Here's how the part is built. I have some questions about the finished solid (model axes, mm). A direction names the side the tool comes from. Coordinates: 2 decimals unless noted, no trailing zeros. Loops run counter-clockwise (first coordinate to the right, second up) from the corner with the lowest first, then second, coordinate; pieces in that order, holes last.
from build123d import *

# Parameters (mm, degrees)
SKETCH1_R           = 2.55
BOSS_EXTRUDE1_DEPTH = 8
SKETCH2_R           = 3.175
CUT_EXTRUDE1_DEPTH  = 1
CUT_EXTRUDE2_START  = -1
SKETCH3_R           = 3.175
CUT_EXTRUDE2_DEPTH  = 1
BOSS_EXTRUDE2_DEPTH = 8
SKETCH5_W           = 8
SKETCH5_H           = 56
BOSS_EXTRUDE3_DEPTH = 8
SKETCH6_W           = 4
SKETCH6_H           = 24
CUT_EXTRUDE3_DEPTH  = 8
FILLET2_R           = 4
SKETCH7_R           = 2.55
CUT_EXTRUDE4_DEPTH  = 8
SKETCH8_R           = 3.175
CUT_EXTRUDE5_DEPTH  = 1
CUT_EXTRUDE6_START  = -1
SKETCH9_R           = 3.175
CUT_EXTRUDE6_DEPTH  = 1
FILLET3_R           = 4
FILLET5_R           = 4


# Some blends are built 0.0001 mm under size
with BuildPart() as part:
    # Sketch1 → Boss-Extrude1 (new body)
    with BuildSketch(Plane.YZ):
        Polygon((0, 0), (72, 0), (72, 24), (88, 24), (88, 32), (64, 32), (64, 8), (0, 8), align=None)
        with Locations(Location((12, 4, 0), (0, 0, 270))):
            Circle(SKETCH1_R, mode=Mode.SUBTRACT)
        with Locations(Location((44, 4, 0), (0, 0, 270))):
            Circle(SKETCH1_R, mode=Mode.SUBTRACT)
        with Locations(Location((60, 4, 0), (0, 0, 270))):
            Circle(SKETCH1_R, mode=Mode.SUBTRACT)
        with Locations(Location((68, 28, 0), (0, 0, 270))):
            Circle(SKETCH1_R, mode=Mode.SUBTRACT)
        with Locations(Location((84, 28, 0), (0, 0, 270))):
            Circle(SKETCH1_R, mode=Mode.SUBTRACT)
    extrude(amount=BOSS_EXTRUDE1_DEPTH)

    # Sketch2 → Cut-Extrude1 (cut)
    with BuildSketch(Plane.YZ.offset(8)):
        with Locations(Location((68, 28, 0), (0, 0, 270))):
            Circle(SKETCH2_R)
        with Locations(Location((84, 28, 0), (0, 0, 270))):
            Circle(SKETCH2_R)
        with Locations(Location((12, 4, 0), (0, 0, 270))):
            Circle(SKETCH2_R)
        with Locations(Location((44, 4, 0), (0, 0, 270))):
            Circle(SKETCH2_R)
        with Locations(Location((60, 4, 0), (0, 0, 270))):
            Circle(SKETCH2_R)
    extrude(amount=-CUT_EXTRUDE1_DEPTH, mode=Mode.SUBTRACT)

    # Sketch3 → Cut-Extrude2 (cut)
    with BuildSketch(Plane(origin=(0, 0, 0), x_dir=(0, -1, 0), z_dir=(-1, 0, 0)).offset(CUT_EXTRUDE2_START)):
        with Locations(Location((-12, 4, 0), (0, 0, 270))):
            Circle(SKETCH3_R)
        with Locations(Location((-84, 28, 0), (0, 0, 270))):
            Circle(SKETCH3_R)
        with Locations(Location((-68, 28, 0), (0, 0, 270))):
            Circle(SKETCH3_R)
        with Locations(Location((-60, 4, 0), (0, 0, 270))):
            Circle(SKETCH3_R)
        with Locations(Location((-44, 4, 0), (0, 0, 270))):
            Circle(SKETCH3_R)
    extrude(amount=CUT_EXTRUDE2_DEPTH, mode=Mode.SUBTRACT)

    # Sketch4 → Boss-Extrude2 (add)
    with BuildSketch(Plane.XY.offset(8)):
        with BuildLine():
            Line((0, 0), (0, -4))
            ThreePointArc((0, -4), (0.723391823, -6.294305745), (2.631919427, -7.758770483))
            Line((2.631919427, -7.758770483), (15.787616118, -12.54705249))
            Line((15.787616118, -12.54705249), (18.523777264, -5.029511523))
            Line((18.523777264, -5.029511523), (8, -1.199169847))
            Line((8, -1.199169847), (8, 0))
            Line((8, 0), (0, 0))
        make_face()
    extrude(amount=-BOSS_EXTRUDE2_DEPTH)

    # Sketch5 → Boss-Extrude3 (add)
    with BuildSketch(Plane(origin=(0.550416468, 1.512256816, 0), x_dir=(-0.9396926207859096, 0.34202014332566544, 0), z_dir=(0.3420201433256654, 0.9396926207859095, 0))):
        with Locations((-15.126851056, -4)):
            Rectangle(SKETCH5_W, SKETCH5_H)
    extrude(amount=-BOSS_EXTRUDE3_DEPTH)

    # Sketch6 → Cut-Extrude3 (cut)
    with BuildSketch(Plane(origin=(0.550416468, 1.512256816, 0), x_dir=(-0.9396926207859096, 0.34202014332566544, 0), z_dir=(0.3420201433256654, 0.9396926207859095, 0))):
        with Locations((-17.126851056, -4)):
            Rectangle(SKETCH6_W, SKETCH6_H)
    extrude(amount=-CUT_EXTRUDE3_DEPTH, mode=Mode.SUBTRACT)

    # Fillet2
    # the kernel refuses this fillet: 4 mm, written as the material it adds along each edge
    with BuildSketch(Plane(origin=(8.270075151, -9.810891343, 0), x_dir=(-0.9396926207859096, 0.34202014332566544, 0), z_dir=(0.34202014332566544, 0.9396926207859096, 0))) as fillet2_piece_1_section:
        with BuildLine():
            CenterArc((FILLET2_R, -FILLET2_R), FILLET2_R, 90, 90)
            Line((0, -FILLET2_R), (0, 0))
            Line((0, 0), (FILLET2_R, 0))
        make_face()
    fillet2_piece_1 = extrude(amount=8, mode=Mode.PRIVATE)
    fillet2_piece_1 = split(fillet2_piece_1, bisect_by=Plane(origin=(8, -7.10901072, -0.334730566), z_dir=(-1, 0, 0)), keep=Keep.TOP, mode=Mode.PRIVATE)
    add(fillet2_piece_1)
    with BuildSketch(Plane(origin=(8.270075151, -9.810891343, 0), x_dir=(-0.9396926207859096, 0.34202014332566544, 0), z_dir=(0.34202014332566544, 0.9396926207859096, 0))) as fillet2_piece_2_section:
        with BuildLine():
            CenterArc((FILLET2_R, -FILLET2_R), FILLET2_R, 90, 90)
            Line((0, -FILLET2_R), (0, 0))
            Line((0, 0), (FILLET2_R, 0))
        make_face()
    fillet2_piece_2 = extrude(amount=8, mode=Mode.PRIVATE)
    fillet2_piece_2 = split(fillet2_piece_2, bisect_by=Plane(origin=(8, -5.333791146, -1.076258135), z_dir=(1, 0, 0)), keep=Keep.TOP, mode=Mode.PRIVATE)
    add(fillet2_piece_2)
    with BuildSketch(Plane(origin=(8.270075151, -9.810891343, 0), x_dir=(-0.9396926207859096, 0.34202014332566544, 0), z_dir=(0.34202014332566544, 0.9396926207859096, 0))) as fillet2_piece_3_section:
        with BuildLine():
            CenterArc((FILLET2_R, -FILLET2_R), FILLET2_R, 90, 90)
            Line((0, -FILLET2_R), (0, 0))
            Line((0, 0), (FILLET2_R, 0))
        make_face()
    fillet2_piece_3 = extrude(amount=18, mode=Mode.PRIVATE)
    fillet2_piece_3 = split(fillet2_piece_3, bisect_by=Plane(origin=(7.527179325, -1.027077195, 0.031937464), z_dir=(0.3420201433256657, 0.9396926207859095, 0)), keep=Keep.TOP, mode=Mode.PRIVATE)
    fillet2_piece_3 = split(fillet2_piece_3, bisect_by=Plane(origin=(8, -0.377545132, 0.031937464), z_dir=(-1, 0, 0)), keep=Keep.TOP, mode=Mode.PRIVATE)
    add(fillet2_piece_3)
    with BuildSketch(Plane(origin=(11.006236298, -2.293350377, 8), x_dir=(-0.9396926207859096, 0.3420201433256654, 0), z_dir=(-0.34202014332566544, -0.9396926207859096, 0))) as fillet2_piece_4_section:
        with BuildLine():
            CenterArc((FILLET2_R, -FILLET2_R), FILLET2_R, 90, 90)
            Line((0, -FILLET2_R), (0, 0))
            Line((0, 0), (FILLET2_R, 0))
        make_face()
    fillet2_piece_4 = extrude(amount=8, mode=Mode.PRIVATE)
    fillet2_piece_4 = split(fillet2_piece_4, bisect_by=Plane(origin=(8, -5.333791146, 9.076258135), z_dir=(1, 0, 0)), keep=Keep.TOP, mode=Mode.PRIVATE)
    add(fillet2_piece_4)
    with BuildSketch(Plane(origin=(14.426437731, 7.103575831, 8), x_dir=(-0.9396926207859096, 0.34202014332566544, 0), z_dir=(-0.34202014332566544, -0.9396926207859096, 0))) as fillet2_piece_5_section:
        with BuildLine():
            CenterArc((FILLET2_R, -FILLET2_R), FILLET2_R, 90, 90)
            Line((0, -FILLET2_R), (0, 0))
            Line((0, 0), (FILLET2_R, 0))
        make_face()
    fillet2_piece_5 = extrude(amount=18, mode=Mode.PRIVATE)
    fillet2_piece_5 = split(fillet2_piece_5, bisect_by=Plane(origin=(7.527179325, -1.027077195, 7.968062536), z_dir=(0.3420201433256657, 0.9396926207859095, 0)), keep=Keep.TOP, mode=Mode.PRIVATE)
    fillet2_piece_5 = split(fillet2_piece_5, bisect_by=Plane(origin=(8, -0.377545132, 7.968062536), z_dir=(-1, 0, 0)), keep=Keep.TOP, mode=Mode.PRIVATE)
    add(fillet2_piece_5)
    with BuildSketch(Plane(origin=(11.006236298, -2.293350377, 8), x_dir=(-0.9396926207859096, 0.3420201433256654, 0), z_dir=(-0.34202014332566544, -0.9396926207859096, 0))) as fillet2_piece_6_section:
        with BuildLine():
            CenterArc((FILLET2_R, -FILLET2_R), FILLET2_R, 90, 90)
            Line((0, -FILLET2_R), (0, 0))
            Line((0, 0), (FILLET2_R, 0))
        make_face()
    fillet2_piece_6 = extrude(amount=8, mode=Mode.PRIVATE)
    fillet2_piece_6 = split(fillet2_piece_6, bisect_by=Plane(origin=(8, -7.10901072, 8.334730566), z_dir=(-1, 0, 0)), keep=Keep.TOP, mode=Mode.PRIVATE)
    add(fillet2_piece_6)
    with BuildSketch(Plane(origin=(14.765006781, -3.66143095, -16), x_dir=(0, 0, 1), z_dir=(-0.34202014332566544, -0.9396926207859096, 0)), Plane(origin=(14.765006781, -3.66143095, 8), x_dir=(0.9396926207859096, -0.34202014332566544, 0), z_dir=(-0.34202014332566544, -0.9396926207859096, 0))) as fillet2_piece_7:
        with BuildLine():
            CenterArc((FILLET2_R, -FILLET2_R), FILLET2_R, 90, 90)
            Line((0, -FILLET2_R), (0, 0))
            Line((0, 0), (FILLET2_R, 0))
        make_face()
    extrude(amount=8)
    # the kernel refuses this fillet: 4 mm, written as the material it takes off along each edge
    with BuildSketch(Plane(origin=(1.60931009, 1.126851056, -32), x_dir=(-0.3420201433256655, -0.9396926207859096, 0), z_dir=(0.9396926207859096, -0.34202014332566544, 0)), Plane(origin=(27.920703472, -8.449712957, 24), x_dir=(-0.34202014332566544, -0.9396926207859096, 0), z_dir=(-0.9396926207859096, 0.34202014332566544, 0))) as fillet2_2_piece_1:
        with BuildLine():
            CenterArc((FILLET2_R, -FILLET2_R), FILLET2_R, 90, 90)
            Line((0, -FILLET2_R), (0, 0))
            Line((0, 0), (FILLET2_R, 0))
        make_face()
    extrude(amount=28, mode=Mode.SUBTRACT)
    with BuildSketch(Plane(origin=(-1.126851056, -6.39068991, -32), x_dir=(0.34202014332566544, 0.9396926207859096, 0), z_dir=(0.9396926207859096, -0.34202014332566544, 0)), Plane(origin=(25.184542326, -15.967253923, 24), x_dir=(0.34202014332566544, 0.9396926207859096, 0), z_dir=(-0.9396926207859096, 0.34202014332566544, 0))) as fillet2_2_piece_2:
        with BuildLine():
            CenterArc((FILLET2_R, FILLET2_R), FILLET2_R, 180, 90)
            Line((0, FILLET2_R), (0, 0))
            Line((0, 0), (FILLET2_R, 0))
        make_face()
    extrude(amount=28, mode=Mode.SUBTRACT)

    # Sketch7 → Cut-Extrude4 (cut)
    with BuildSketch(Plane(origin=(17.973360797, -6.54176834, 0), x_dir=(0.3420201433256649, 0.9396926207859099, 0), z_dir=(0.9396926207859099, -0.3420201433256649, 0))):
        with Locations((-2.39068991, 20)):
            Circle(SKETCH7_R)
        with Locations((-2.39068991, -28)):
            Circle(SKETCH7_R)
    extrude(amount=-CUT_EXTRUDE4_DEPTH, mode=Mode.SUBTRACT)

    # Sketch8 → Cut-Extrude5 (cut)
    with BuildSketch(Plane(origin=(17.973360797, -6.54176834, 0), x_dir=(0.3420201433256649, 0.9396926207859099, 0), z_dir=(0.9396926207859099, -0.3420201433256649, 0))):
        with Locations((-2.39068991, 20)):
            Circle(SKETCH8_R)
        with Locations((-2.39068991, -28)):
            Circle(SKETCH8_R)
    extrude(amount=-CUT_EXTRUDE5_DEPTH, mode=Mode.SUBTRACT)

    # Sketch9 → Cut-Extrude6 (cut)
    with BuildSketch(Plane(origin=(10.45581983, -3.805607193, 0), x_dir=(-0.3420201433256654, -0.9396926207859095, 0), z_dir=(-0.9396926207859095, 0.3420201433256654, 0)).offset(CUT_EXTRUDE6_START)):
        with Locations(Location((2.39068991, -28, 0), (0, 0, 180))):
            Circle(SKETCH9_R)
        with Locations(Location((2.39068991, 20, 0), (0, 0, 180))):
            Circle(SKETCH9_R)
    extrude(amount=CUT_EXTRUDE6_DEPTH, mode=Mode.SUBTRACT)

    # Fillet3
    fillet3_edges = [part.edges().sort_by_distance(p)[0] for p in [
        (4, 72, 0),
        (4, 64, 8),
    ]]
    fillet(fillet3_edges, radius=FILLET3_R)

    # Fillet5
    fillet5_edges = [part.edges().sort_by_distance(p)[0] for p in [
        (4, 88, 24),
        (4, 64, 32),
        (4, 88, 32),
    ]]
    fillet(fillet5_edges, radius=FILLET5_R - 0.0001)  # a hair under: the kernel refuses the full size


solid = part.part
Q1. For faces 1 (the cylindrical face through (4.056, 62.797, 9.141)), 2 (the cylindrical face through (0.51, 47.1, 4.69)), 3 (the flat face through (13.416, -7.368, -4.112)), 4 (the cylindrical face through (3.958, 68.112, 30.548)), which set-ups out of +Z, -Z, +X, -X, +Y, -Y let a thin tool reach every point of the face, with its end or its side?
Q2. Will these pins go through, and if not, where does the flat tip stop? P1, Ø9, axis at x = 3.5, y = 80.5, coming from the -Z side; P2, Ø4, axis at y = 44, z = 4, coming from the -X side; P3, Ø5, axis at y = 13.5, z = 3, coming from the +X side; P4, Ø5, axis at x = 8.5, y = 10.5, coming from the -Z side.
Q3. Suppose I cut it at A-A on y = 44. Write out the boundary of the cut face in (x, z) (3 decimals), and give its area (3 significant figures).
Q4. Please list where these lines run through material, in increasing order: probe 1 along Y at (x, z) = (2.8, 28); probe 2 along Y at (x, z) = (3.55, 4); probe 3 along Y at (x, z) = (0.8, 4) (3 decimals).
Q5. Suppose I cut it at C-C on z = -18. Write out the boundary of the cut face in (x, y), and give its area (3 significant figures).
Q6. We'd pull the mould along Z, two halves only. Please class faces 5 (the flat face through (9.657, -5.999, -15.085)), 6 (the cylindrical face through (4.056, 86.797, 30.859)), 7 (the cylindrical face through (0.51, 80.85, 28.41)): pulls with the +Z half, pulls with the -Z half, needs draft (parallel to the pull), parting line crosses it, or undercut.
Q7. Suppose I cut it at B-B on y = 13.5. Write out the boundary of the cut face in (x, z).
Check values:
1. face 1: +Z, +X, -X
1. face 2: -X
1. face 3: +X, -Y
1. face 4: +X, -X
2. P1: stops at z = 24
2. P2: passes through
2. P3: stops at x = 8
2. P4: stops at z = 0
3. outline: (0, 0) - (8, 0) - (8, 0.825) - (7, 0.825) - (7, 1.45) - (1, 1.45) - (1, 0.825) - (0, 0.825) - close; (0, 7.175) - (1, 7.175) - (1, 6.55) - (7, 6.55) - (7, 7.175) - (8, 7.175) - (8, 8) - (0, 8) - close
3. area: 20.7 mm2
4. probe 1: y = 64 to 65.45, 70.55 to 81.45, 86.55 to 88
4. probe 2: y = -8.09 to 9.45, 14.55 to 41.45, 46.55 to 57.45, 62.55 to 72
4. probe 3: y = -6.4 to 8.825, 15.175 to 40.825, 47.175 to 56.825, 63.175 to 72
5. outline: (8.27, -9.81) - (15.79, -12.55) - (18.52, -5.03) - (11.01, -2.29) - close
5. area: 64.0 mm2
6. face 5: needs draft
6. face 6: pulls with the +Z half
6. face 7: undercut
7. outline: (0, 0) - (8, 0) - (8, 1.2) - (7, 1.2) - (7, 1.94) - (1, 1.94) - (1, 1.2) - (0, 1.2) - close; (0, 6.8) - (1, 6.8) - (1, 6.06) - (7, 6.06) - (7, 6.8) - (8, 6.8) - (8, 8) - (0, 8) - close
